from build123d import *

# Parameters (mm, degrees)
SKETCH1_W           = 48
SKETCH1_H           = 80
BOSS_EXTRUDE1_DEPTH = 5


with BuildPart() as part:
    # Sketch1 → Boss-Extrude1 (new body)
    with BuildSketch(Plane.XY):
        Polygon((25.508982036, 41.676646707), (-22.491017964, 41.676646707), (-34.491017964, 10.002955871), (-34.491017964, 1.676646707), (-22.491017964, 1.676646707), (25.508982036, 1.676646707), align=None)
        Polygon((73.508982036, 41.676646707), (25.508982036, 41.676646707), (25.508982036, 1.676646707), (73.508982036, 1.676646707), (85.508982036, 1.676646707), (85.508982036, 10.002955871), align=None)
        with Locations((1.508982036, -38.323353293)):
            Rectangle(SKETCH1_W, SKETCH1_H)
        with Locations((49.508982036, -38.323353293)):
            Rectangle(SKETCH1_W, SKETCH1_H)
        Polygon((25.508982036, -98.323353293), (25.508982036, -78.323353293), (-22.491017964, -78.323353293), (10.508982036, -98.323353293), align=None)
        Polygon((73.508982036, -78.323353293), (25.508982036, -78.323353293), (25.508982036, -98.323353293), (40.508982036, -98.323353293), align=None)
    extrude(amount=BOSS_EXTRUDE1_DEPTH)


solid = part.part
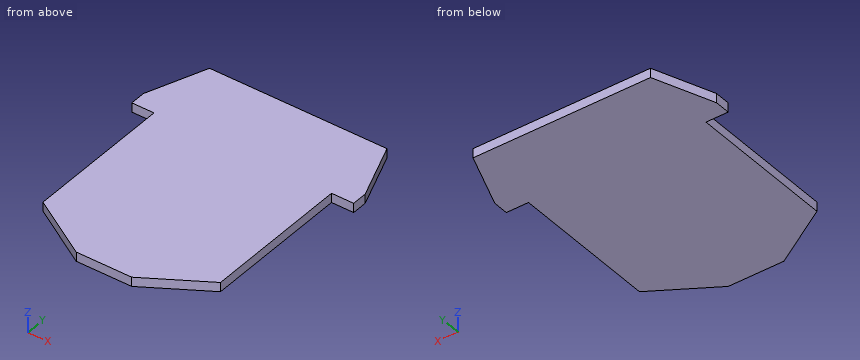
Source: CAD feature listing. Evaluate the final solid. Frame: model axes, mm. Coordinates: 2 decimals unless noted, no trailing zeros. Loops run counter-clockwise (first coordinate to the right, second up) from the corner with the lowest first, then second, coordinate; pieces in that order, holes last. Notation, with made-up numbers: (53, 15) -> (99, 15) arc R33 cw to (99, 50) -> close; hole circle Ø2 at (48, 34). An arc over 180 degrees is marked (long way). Answer in a Markdown table with one row per item. Add a question column.
Q1. Section A-A on z = 2.6. Return the cut outline in (x, y), and give its area (3 significant figures).
Q2. Ray query, line 1 along X through (y, z) = (-15, 0.4); line 2 along X through (y, z) = (18, 2.9); line 3 along Y through (x, z) = (62.5, 0.3). Return the intervals inside material, ascending.
Q3. Section B-B on y = -7. Return the cut outline in (x, z), and give its area (3 significant figures).
Q4. Contact query for flat-ended pins moving along their axis: pin 1 Ø2.5 at (y, z) = (-45, 1.5) entering from -X; pin 2 Ø4 at (x, y) = (39, -12.5) entering from -Z; pin 3 Ø1.5 at (y, z) = (-25.5, 1.5) entering from +X. Output: stop coordinate, or through.
Q5. Section C-C on x = 78.5. Return the cut outline in (y, z).
Computed values:
| question | item | result |
|---|---|---|
| 1 | outline | (-34.49, 1.68) -> (-22.49, 1.68) -> (-22.49, -78.32) -> (10.51, -98.32) -> (40.51, -98.32) -> (73.51, -78.32) -> (73.51, 1.68) -> (85.51, 1.68) -> (85.51, 10) -> (73.51, 41.68) -> (-22.49, 41.68) -> (-34.49, 10) -> close |
| 1 | area | 13,400 mm^2 |
| 2 | line 1 | x = -22.49 to 73.51 |
| 2 | line 2 | x = -31.46 to 82.48 |
| 2 | line 3 | y = -85 to 41.68 |
| 3 | outline | (-22.49, 0) -> (73.51, 0) -> (73.51, 5) -> (-22.49, 5) -> close |
| 3 | area | 480 mm^2 |
| 4 | pin 1 | stops at x = -22.49 |
| 4 | pin 2 | stops at z = 0 |
| 4 | pin 3 | stops at x = 73.51 |
| 5 | outline | (1.68, 0) -> (28.5, 0) -> (28.5, 5) -> (1.68, 5) -> close |
